```python
from build123d import *

# Parameters (mm, degrees)
SKETCH_1_R               = 14
SKETCH_1_R_2             = 1.5
SKETCH_1_R_3             = 3
EXTRUDE_1_DEPTH          = 4
SKETCH_3_R               = 7.5
SKETCH_3_R_2             = 3
EXTRUDE_2_DEPTH          = 12
SKETCH_4_R               = 1.5
CUT_EXTRUDE_1_DEPTH      = 15
CUT_EXTRUDE_1_DEPTH_BACK = 15


with BuildPart() as part:
    # ｽｹｯﾁ1 → ﾎﾞｽ - 押し出し1 (new body)
    with BuildSketch(Plane.XY):
        Circle(SKETCH_1_R)
        with Locations((-10.5, 0)):
            Circle(SKETCH_1_R_2, mode=Mode.SUBTRACT)
        with Locations((5.25, -9.09326674)):
            Circle(SKETCH_1_R_2, mode=Mode.SUBTRACT)
        with Locations((5.25, 9.09326674)):
            Circle(SKETCH_1_R_2, mode=Mode.SUBTRACT)
        Circle(SKETCH_1_R_3, mode=Mode.SUBTRACT)
    extrude(amount=EXTRUDE_1_DEPTH)

    # ｽｹｯﾁ3 → ﾎﾞｽ - 押し出し2 (add)
    with BuildSketch(Plane.XY.offset(4)):
        Circle(SKETCH_3_R)
        Circle(SKETCH_3_R_2, mode=Mode.SUBTRACT)
    extrude(amount=EXTRUDE_2_DEPTH)

    # ｽｹｯﾁ4 → ｶｯﾄ - 押し出し1 (cut, two sides)
    with BuildSketch(Plane(origin=(0, 0, 0), x_dir=(1, 0, 0), z_dir=(0, 1, 0))) as cut_extrude_1_sk:
        with Locations((0, -8)):
            Circle(SKETCH_4_R)
    extrude(amount=CUT_EXTRUDE_1_DEPTH, mode=Mode.SUBTRACT)
    extrude(cut_extrude_1_sk.sketch, amount=-CUT_EXTRUDE_1_DEPTH_BACK, mode=Mode.SUBTRACT)


solid = part.part
```
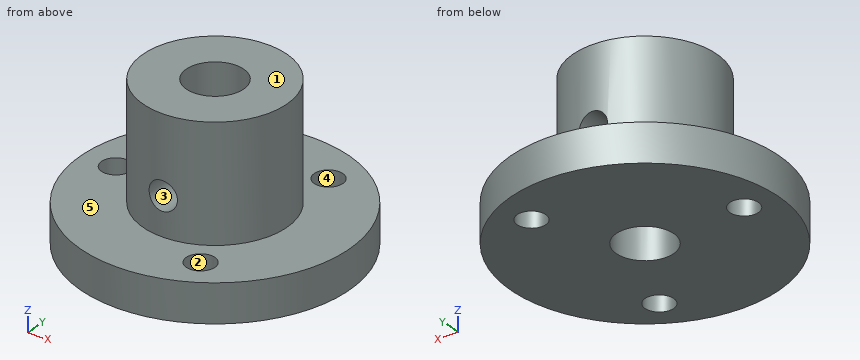
Here's how the part is built. I have some questions about the finished solid (model axes, mm). Face numbers are marked on the shaded views. A direction names the side the tool comes from. Coordinates: 2 decimals unless noted, no trailing zeros. Loops run counter-clockwise (first coordinate to the right, second up) from the corner with the lowest first, then second, coordinate; pieces in that order, holes last. Notation, with made-up numbers: (-11, -40) - (37, -40) arc R24 cw to (37, -18) - close; hole circle Ø2 at (66, -9). An arc over 180 degrees is marked (long way). Answer as CSV lines item,"result".
Q1. We'd pull the mould along Z, two halves only. Please class the marked faces 1, 2 and 3: pulls with the +Z half, pulls with the -Z half, needs draft (parallel to the pull), parting line crosses it, or undercut.
Response:
face 1,"pulls with the +Z half"
face 2,"needs draft"
face 3,"undercut"
Q2. If we section it at A-A, the plane y = 0: Write out the boundary of the cut face in (x, z).
Response:
outline,"(-14, 0) - (-12, 0) - (-12, 4) - (-14, 4) - close; (-9, 0) - (-3, 0) - (-3, 16) - (-7.5, 16) - (-7.5, 4) - (-9, 4) - close; (3, 0) - (14, 0) - (14, 4) - (7.5, 4) - (7.5, 16) - (3, 16) - close"
Q3. If we section it at D-D, the plane z = 4.5: Write out the boundary of the cut face in (x, y), and give its area (3 significant figures).
Response:
outline,"circle Ø15 at (0, 0); hole circle Ø6 at (0, 0)"
area,"148 mm2"
Q4. If I drill on L1, parallel to Y at x = 5.25, z = 2.7; L2, parallel to Z at x = 0, y = -5.6; L3, parallel to Z at x = 8.5, y = -2.5, over which ranges is the centre line in solid material (lowest first)? Write a range as [from, to].
Response:
L1,"[-12.98, -10.59], [-7.59, 7.59], [10.59, 12.98]"
L2,"[0, 6.5], [9.5, 16]"
L3,"[0, 4]"
Q5. For the marked faces 4 and 5, which set-ups out of +Z, -Z, +X, -X, +Y, -Y let a thin tool reach every point of the face, with its end or its side?
Response:
face 4,"+Z, -Z"
face 5,"+Z"
Q6. If we section it at C-C, the plane x = 5.25: Write out the boundary of the cut face in (y, z), and give its area (3 significant figures).
Response:
outline,"(-12.98, 0) - (-10.59, 0) - (-10.59, 4) - (-12.98, 4) - close; (-7.59, 0) - (7.59, 0) - (7.59, 4) - (5.36, 4) - (5.36, 16) - (-5.36, 16) - (-5.36, 4) - (-7.59, 4) - close; (10.59, 0) - (12.98, 0) - (12.98, 4) - (10.59, 4) - close"
area,"208 mm2"
Q7. For pin 1 (2.5 mm diameter, centred on x = 0, z = 8, fed in from -Y); pin 2 (8 mm diameter, centred on x = -3, z = 11.5, fed in from +Y); pin 3 (5 mm diameter, centred on x = 5.25, y = 9.09, fed in from +Z); pin 4 (1.5 mm diameter, centred on x = 7.5, z = 7, fed in from +Y), each with a flat end and sliding along its axis, tell me the tip position at first contact or that it passes through.
Response:
pin 1,"through"
pin 2,"y = 7.5"
pin 3,"z = 4"
pin 4,"y = 3.27"
Q8. If we section it at B-B, the plane x = 0: Write out the boundary of the cut face in (y, z).
Response:
outline,"(-14, 0) - (-3, 0) - (-3, 6.5) - (-7.5, 6.5) - (-7.5, 4) - (-14, 4) - close; (-7.5, 9.5) - (-3, 9.5) - (-3, 16) - (-7.5, 16) - close; (3, 0) - (14, 0) - (14, 4) - (7.5, 4) - (7.5, 6.5) - (3, 6.5) - close; (3, 9.5) - (7.5, 9.5) - (7.5, 16) - (3, 16) - close"
